The model under review builds one solid part; all positions refer to its coordinate system, in mm. Coordinates: 2 decimals unless noted, no trailing zeros. Write each loop counter-clockwise with the first axis right and the second up, starting at its lowest first coordinate (ties: lowest second). Pieces come first, ordered by that corner, then holes. Notation, with made-up numbers: (-34, 29.25) - (-14, 29.25) arc R28 cw to (-14, 49.25) - close; hole circle Ø9 at (-23, 75.25). An arc over 180 degrees is marked (long way). Return JSON: item names as keys, results as strings. Group by question number.
(1) We need section B-B on z = 3.7. Give the number of separate pieces and of enclosed holes in the cut face, then the cut area to 3 significant figures.
(2) We need section C-C on x = 16. State the section outline as (y, z) points.
(3) We need section D-D on y = -42.5. State the section outline as (x, z) points, then the cut area to 4 significant figures.
(4) We need section A-A on y = -4. State the section outline as (x, z) points.
(5) For pin 1 Ø1.3 at (x, z) = (-70, 2.5) entering from -Y; pin 2 Ø1.3 at (x, z) = (-88.5, 1.5) entering from -Y; pin 3 Ø1.3 at (x, z) = (-70.5, 2.5) entering from +Y, all flat-tipped, find the tip position at first contact; note any pin that passes through.
(6) To check wall thickness, follow L1, parallel to X at y = 43, z = 3.45; L2, parallel to X at y = 47, z = 1.7; L3, parallel to X at y = -29, z = 2. State the ranges of each line that lie inside material, in increasing order. Write a range as from..to.
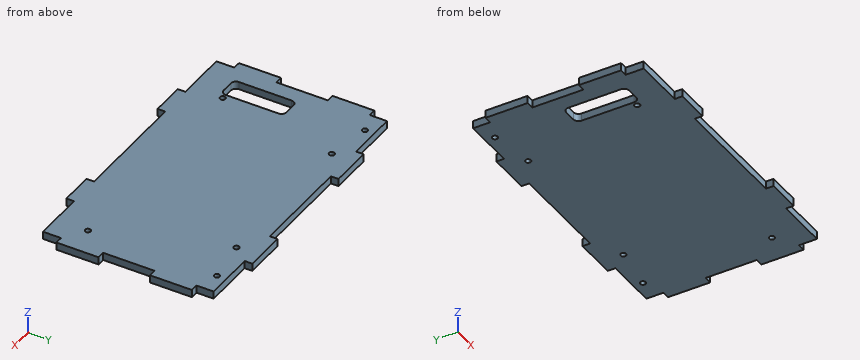
Autodesk Fusion 360 part; units mm, degrees
sketch "Sketch1" plane through (0, 0, 0) normal (0, 0, 1) x (1, 0, 0)
  line L0 (90, -52.5) -> (-90, -52.5)
  line L1 (-90, -52.5) -> (-90, 52.5)
  line L2 (-90, 52.5) -> (90, 52.5)
  line L3 (90, 52.5) -> (90, -52.5)
  line L4 (90, -52.5) -> (-90, 52.5) construction
  line L5 (-90, -52.5) -> (90, 52.5) construction
  line L6 (-85.5, 52.5) -> (-85.5, -52.5)
  line L7 (85.5, 52.5) -> (85.5, -52.5)
  line L8 (-90, -48) -> (90, -48)
  line L9 (-90, -52.5) -> (-55, -52.5)
  line L10 (-55, -52.5) -> (-55, -48)
  line L11 (-55, -48) -> (-90, -48)
  line L12 (-90, -48) -> (-90, -52.5)
  line L13 (-55, -52.5) -> (-35, -52.5)
  line L14 (-35, -52.5) -> (-35, -48)
  line L15 (-35, -48) -> (-55, -48)
  line L16 (-55, -48) -> (-55, -52.5)
  line L17 (90, -52.5) -> (55, -52.5)
  line L18 (55, -52.5) -> (55, -48)
  line L19 (55, -48) -> (90, -48)
  line L20 (90, -48) -> (90, -52.5)
  line L21 (-90, -52.5) -> (-85.5, -52.5)
  line L22 (-85.5, -52.5) -> (-85.5, -37.5)
  line L23 (-85.5, -37.5) -> (-90, -37.5)
  line L24 (-90, -37.5) -> (-90, -52.5)
  line L25 (90, -52.5) -> (85.5, -52.5)
  line L26 (85.5, -52.5) -> (85.5, -37.5)
  line L27 (85.5, -37.5) -> (90, -37.5)
  line L28 (90, -37.5) -> (90, -52.5)
  line L29 (-85.5, -37.5) -> (-90, -37.5)
  line L30 (-90, -37.5) -> (-90, -12.5)
  line L31 (-90, -12.5) -> (-85.5, -12.5)
  line L32 (-85.5, -12.5) -> (-85.5, -37.5)
  line L33 (90, -37.5) -> (85.5, -37.5)
  line L34 (85.5, -37.5) -> (85.5, -12.5)
  line L35 (85.5, -12.5) -> (90, -12.5)
  line L36 (90, -12.5) -> (90, -37.5)
  line L37 (-85.5, -12.5) -> (-90, -12.5)
  line L38 (-90, -12.5) -> (-90, 17.5)
  line L39 (-90, 17.5) -> (-85.5, 17.5)
  line L40 (-85.5, 17.5) -> (-85.5, -12.5)
  line L41 (-85.5, 17.5) -> (-90, 17.5)
  line L42 (-90, 17.5) -> (-90, 42.5)
  line L43 (-90, 42.5) -> (-85.5, 42.5)
  line L44 (-85.5, 42.5) -> (-85.5, 17.5)
  line L45 (90, -12.5) -> (85.5, -12.5)
  line L46 (85.5, -12.5) -> (85.5, 17.5)
  line L47 (85.5, 17.5) -> (90, 17.5)
  line L48 (90, 17.5) -> (90, -12.5)
  line L49 (90, 17.5) -> (85.5, 17.5)
  line L50 (85.5, 17.5) -> (85.5, 42.5)
  line L51 (85.5, 42.5) -> (90, 42.5)
  line L52 (90, 42.5) -> (90, 17.5)
  line L53 (55, -52.5) -> (35, -52.5)
  line L54 (35, -52.5) -> (35, -48)
  line L55 (35, -48) -> (55, -48)
  line L56 (55, -48) -> (55, -52.5)
  line L57 (-90, 43) -> (90, 43) construction
  line L58 (0, 43) -> (0, 40) construction
  circle A0 centre (47, 43) radius 1.6
  circle A1 centre (-47, 43) radius 1.6
  line L59 (-90, 47) -> (90, 47) construction
  circle A2 centre (73, 47) radius 1.6
  circle A3 centre (-73, 47) radius 1.6
  circle A4 centre (73, -29) radius 1.6
  circle A5 centre (-60, -29) radius 1.6
  line L60 (-66, -32) -> (-73, -32)
  line L61 (-76, -29) -> (-76, 2)
  line L62 (-73, 5) -> (-66, 5)
  line L63 (-63, 2) -> (-63, -29)
  line L64 (-63, -32) -> (-76, 5) construction
  line L65 (-76, -32) -> (-63, 5) construction
  arc A6 (-63, 2) -> (-66, 5) centre (-66, 2) ccw
  arc A7 (-73, 5) -> (-76, 2) centre (-73, 2) ccw
  arc A8 (-76, -29) -> (-73, -32) centre (-73, -29) ccw
  arc A9 (-66, -32) -> (-63, -29) centre (-66, -29) ccw
  line L66 (-55, 52.5) -> (-30, 52.5)
  line L67 (-30, 52.5) -> (-30, 57)
  line L68 (-30, 57) -> (-55, 57)
  line L69 (-55, 57) -> (-55, 52.5)
  line L70 (30, 52.5) -> (55, 52.5)
  line L71 (55, 52.5) -> (55, 57)
  line L72 (55, 57) -> (30, 57)
  line L73 (30, 57) -> (30, 52.5)
  point P0 (-69.5, -13.5)
  dimension "d1" = 180
  dimension "d2" = 105
  dimension "d3" = 4.5
  dimension "d4" = 4.5
  dimension "d5" = 4.5
  dimension "d6" = 35
  dimension "d7" = 20
  dimension "d8" = 35
  dimension "d10" = 15
  dimension "d11" = 15
  dimension "d12" = 25
  dimension "d13" = 25
  dimension "d14" = 30
  dimension "d15" = 25
  dimension "d16" = 30
  dimension "d17" = 25
  dimension "d18" = 20
  dimension "d20" = 91
  dimension "d21" = 3.2
  dimension "d22" = 3.2
  dimension "d23" = 47
  dimension "d24" = 47
  dimension "d25" = 4
  dimension "d26" = 3.2
  dimension "d27" = 3.2
  dimension "d28" = 73
  dimension "d29" = 73
  dimension "d30" = 3.2
  dimension "d31" = 72
  dimension "d32" = 3.2
  dimension "d33" = 72
  dimension "d34" = 60
  dimension "d35" = 13
  dimension "d36" = 37
  dimension "d37" = 3
  dimension "d38" = 3
  dimension "d39" = 3
  dimension "d40" = 3
  dimension "d41" = 3
  dimension "d42" = 3
  dimension "d48" = 25
  dimension "d49" = 4.5
  dimension "d50" = 25
  dimension "d51" = 4.5
  dimension "d52" = 35
  dimension "d53" = 35
extrude "Extrude1" add sketch "Sketch1" along normal blind 4.5 contours L0 L8 L18 L53 L54 L55 L56 | L2 L6 L7 L8 L11 L15 L19 L22 L26 L32 L34 L40 L44 L46 L50 L55 L66 L70 | L3 L7 L27 L33 L34 L35 L36 L45 | L0 L8 L10 L13 L14 L15 L16 | L3 L7 L47 L49 L50 L51 L52 | L1 L6 L23 L29 L30 L31 L32 L37 | L2 L70 L71 L72 L73 | L1 L6 L39 L41 L42 L43 L44 | L2 L66 L67 L68 L69
move_face "OffsetFaces1" offset -0.1 4 faces at (55, -51, 1.5) (-35, -51, 1.5) (-30, 54, 1.5) (55, 54, 1.5)
move_face "OffsetFaces2" offset -0.1 4 faces at (35, -51, 1.5) (-55, -51, 1.5) (30, 55.5, 1.5) (-55, 55.5, 1.5)
move_face "OffsetFaces3" offset -0.1 4 faces at (-88.5, 17.5, 1.5) (-87, -37.5, 1.5) (87, -37.5, 1.5) (87, 17.5, 1.5)
move_face "OffsetFaces4" offset -0.1 4 faces at (-88.5, 42.5, 1.5) (-88.5, -12.5, 1.5) (87, 42.5, 1.5) (87, -12.5, 1.5)
equation "TabRelief = -0.1 mm"
equation "d55 = TabRelief"
equation "d56 = TabRelief"
equation "d57 = TabRelief"
equation "d58 = TabRelief"
Ans:
{
 "1": {"separate pieces": "1", "enclosed holes": "7", "area": "17,500 mm²"},
 "2": {"outline": "(-48, 0) - (52.5, 0) - (52.5, 4.5) - (-48, 4.5) - close"},
 "3": {"outline": "(-85.5, 0) - (85.5, 0) - (85.5, 4.5) - (-85.5, 4.5) - close", "area": "769.5 mm²"},
 "4": {"outline": "(-85.5, 0) - (-76, 0) - (-76, 4.5) - (-85.5, 4.5) - close; (-63, 0) - (85.5, 0) - (85.5, 4.5) - (-63, 4.5) - close"},
 "5": {"pin 1": "y = -48", "pin 2": "y = -37.4", "pin 3": "y = 52.5"},
 "6": {"L1": "-85.5..-48.6, -45.4..45.4, 48.6..85.5", "L2": "-85.5..-74.6, -71.4..71.4, 74.6..85.5", "L3": "-90..-76, -63..-61.6, -58.4..71.4, 74.6..90"}
}
